Build history of the part. All positions in model axes, mm. Round coordinates to 2 decimals unless told otherwise and drop trailing zeros. Write each loop counter-clockwise with the first axis right and the second up, starting at its lowest first coordinate (ties: lowest second). Pieces come first, ordered by that corner, then holes. Notation, with made-up numbers: M 35,85 L 62,85 A14 ccw 62,92 Z; hole C -34,63 d10. An arc over 180 degrees is marked long. Use a Markdown table: item, result.
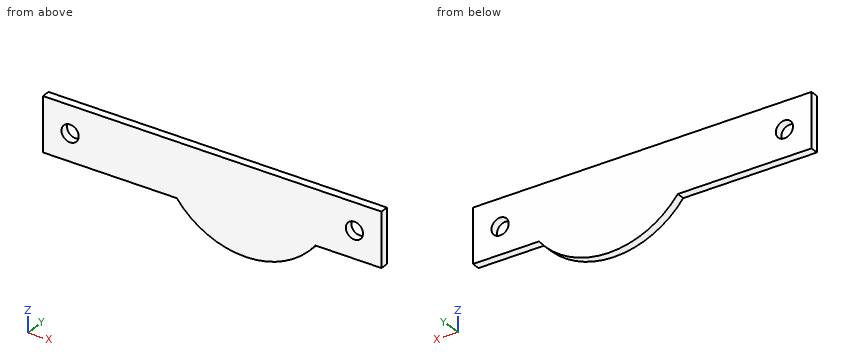
from build123d import *

# Parameters (mm, degrees)
SKETCH_R  = 6.35
PAD_DEPTH = 6


with BuildPart() as part:
    # Sketch → Pad (new body)
    with BuildSketch(Plane.XZ):
        with BuildLine():
            Line((0, 0), (250, 0))
            Line((250, 0), (250, -40))
            Line((250, -40), (201.234754, -40))
            ThreePointArc((98.765246, -40), (150, -65), (201.234754, -40))
            Line((98.765246, -40), (0, -40))
            Line((0, 0), (0, -40))
        make_face()
        with Locations((20, -20)):
            Circle(SKETCH_R, mode=Mode.SUBTRACT)
        with Locations((230, -20)):
            Circle(SKETCH_R, mode=Mode.SUBTRACT)
    extrude(amount=PAD_DEPTH)


solid = part.part
Q1. Cut at A-A on y = -4.1. Give the cut face in (x, z).
Response values:
| item | result |
|---|---|
| outline | M 0,-40 L 98.77,-40 A65 ccw 201.23,-40 L 250,-40 L 250,0 L 0,0 Z; hole C 20,-20 d12.7; hole C 230,-20 d12.7 |
Q2. Cut at D-D on x = 111. Give the cut face in (y, z), and give its area (3 significant figures).
Response values:
| item | result |
|---|---|
| outline | M -6,-52 L 0,-52 L 0,0 L -6,0 Z |
| area | 312 mm2 |
Q3. Drop flat-ended pins along their axis: P1, Ø7.5, axis at x = 230, z = -20, coming from the -Y side; P2, Ø12, axis at x = 181.5, z = -38, coming from the +Y side; P3, Ø3, axis at x = 46, y = -2.5, coming from the -Z side. Give the stop position or say it passes through.
Response values:
| item | result |
|---|---|
| P1 | passes through |
| P2 | stops at y = 0 |
| P3 | stops at z = -40 |
Q4. Drill centre lines: L1, parallel to Z at x = 20, y = -1.9; L2, parallel to X at y = -4.6, z = -21; L3, parallel to X at y = -4.35, z = -15. Where is each one in solid material? Low to high.
Response values:
| item | result |
|---|---|
| L1 | z = -40 to -26.35, -13.65 to 0 |
| L2 | x = 0 to 13.73, 26.27 to 223.73, 236.27 to 250 |
| L3 | x = 0 to 16.09, 23.91 to 226.09, 233.91 to 250 |
Q5. Cut at B-B on x = 230. Give the cut face in (y, z).
Response values:
| item | result |
|---|---|
| outline | M -6,-40 L 0,-40 L 0,-26.35 L -6,-26.35 Z; M -6,-13.65 L 0,-13.65 L 0,0 L -6,0 Z |
Q6. Cut at C-C on z = -20. Give the cut face in (x, y), and give its area (3 significant figures).
Response values:
| item | result |
|---|---|
| outline | M 0,-6 L 13.65,-6 L 13.65,0 L 0,0 Z; M 26.35,-6 L 223.65,-6 L 223.65,0 L 26.35,0 Z; M 236.35,-6 L 250,-6 L 250,0 L 236.35,0 Z |
| area | 1,350 mm2 |
